Source: CAD feature listing. Evaluate the final solid. Frame: model axes, mm. Round coordinates to 2 decimals unless told otherwise and drop trailing zeros. Write each loop counter-clockwise with the first axis right and the second up, starting at its lowest first coordinate (ties: lowest second). Pieces come first, ordered by that corner, then holes. Notation, with made-up numbers: M -23,-30 L -18,-30 A33 cw -18,1 Z; hole C 46,51.25 d3. An arc over 180 degrees is marked long. Answer in a Markdown table with one row per item.
from build123d import *

# Parameters (mm, degrees)
F0_R     = 9.525
F1_DEPTH = 25.4
F3_DEPTH = 25.401
F4_DEPTH = 11.0998
F6_DEPTH = 9.525


with BuildPart() as f1:
    # F0 (on Front) → F1 (new body)
    with BuildSketch(Plane.XZ):
        Circle(F0_R)
    extrude(amount=-F1_DEPTH)

    # F2 (on Front) → F3 (cut, through all)
    with BuildSketch(Plane.XZ):
        with BuildLine():
            ThreePointArc((-4.7625, 0), (-3.367596, -3.367596), (0, -4.7625))
            ThreePointArc((0, -4.7625), (3.367596, -3.367596), (4.7625, 0))
            ThreePointArc((4.7625, 0), (3.367596, 3.367596), (0, 4.7625))
            ThreePointArc((0, 4.7625), (-3.367596, 3.367596), (-4.7625, 0))
        make_face()
    extrude(amount=-F3_DEPTH, mode=Mode.SUBTRACT)

    # F2 (on Front) → F4 (cut)
    with BuildSketch(Plane.XZ):
        with BuildLine():
            Line((0, -4.7625), (4.7625, -4.7625))
            Line((4.7625, -4.7625), (4.7625, 0))
            ThreePointArc((4.7625, 0), (3.367596, -3.367596), (0, -4.7625))
        make_face()
        with BuildLine():
            Line((-4.7625, -4.7625), (0, -4.7625))
            ThreePointArc((0, -4.7625), (-3.367596, -3.367596), (-4.7625, 0))
            Line((-4.7625, 0), (-4.7625, -4.7625))
        make_face()
        with BuildLine():
            ThreePointArc((0, 4.7625), (3.367596, 3.367596), (4.7625, 0))
            Line((4.7625, 0), (4.7625, 4.7625))
            Line((4.7625, 4.7625), (0, 4.7625))
        make_face()
        with BuildLine():
            Line((-4.7625, 4.7625), (-4.7625, 0))
            ThreePointArc((-4.7625, 0), (-3.367596, 3.367596), (0, 4.7625))
            Line((0, 4.7625), (-4.7625, 4.7625))
        make_face()
    extrude(amount=-F4_DEPTH, mode=Mode.SUBTRACT)

    # F5 (on Front) → F6 (cut)
    with BuildSketch(Plane.XZ):
        Polygon((3.65125, -6.324151), (7.3025, 0), (3.65125, 6.324151), (-3.65125, 6.324151), (-7.3025, 0), (-3.65125, -6.324151), align=None)
    extrude(amount=-F6_DEPTH, mode=Mode.SUBTRACT)


solid = f1.part
Q1. Pull-direction query (Z, two-part tool) for faces 1 (the cylindrical face through (-7.559, 12.522, -5.796)), 2 (the flat face through (-4.4, 25.4, 2.3)), 3 (the flat face through (6.05, 4.7, 2.17)); classes: pulls with the +Z half, pulls with the -Z half, needs draft (parallel to the pull), parting line crosses it, or undercut.
Solutions:
| item | result |
|---|---|
| face 1 | parting line crosses it |
| face 2 | needs draft |
| face 3 | undercut |
Q2. Section B-B (x = -2.25). Return loops of the section in (y, z) (1 decimal).
Solutions:
| item | result |
|---|---|
| outline | M 0,-9.3 L 25.4,-9.3 L 25.4,-4.2 L 11.1,-4.2 L 11.1,-4.8 L 9.5,-4.8 L 9.5,-6.3 L 0,-6.3 Z; M 0,6.3 L 9.5,6.3 L 9.5,4.8 L 11.1,4.8 L 11.1,4.2 L 25.4,4.2 L 25.4,9.3 L 0,9.3 Z |
Q3. Material intervals for probe 1 along Y at (x, z) = (-2, -6.25) (3 decimals); probe 2 along Z at (x, y) = (4, 4.5); probe 3 along Z at (x, y) = (-4.5, 9.25), sorted ascending.
Solutions:
| item | result |
|---|---|
| probe 1 | y = 9.525 to 25.4 |
| probe 2 | z = -8.64 to -5.72, 5.72 to 8.64 |
| probe 3 | z = -8.39 to -4.85, 4.85 to 8.39 |
Q4. Contact query for flat-ended pins moving along their axis: pin 1 Ø3 at (y, z) = (18, -5) entering from -X; pin 2 Ø5 at (y, z) = (13, -5.5) entering from -X; pin 3 Ø2.5 at (x, z) = (2, -2.5) entering from -Y; pin 4 Ø1.5 at (x, z) = (-4.5, 0) entering from -Y (3 decimals). Output: stop coordinate, or through.
Solutions:
| item | result |
|---|---|
| pin 1 | stops at x = -8.86 |
| pin 2 | stops at x = -9.04 |
| pin 3 | passes through |
| pin 4 | stops at y = 9.525 |
